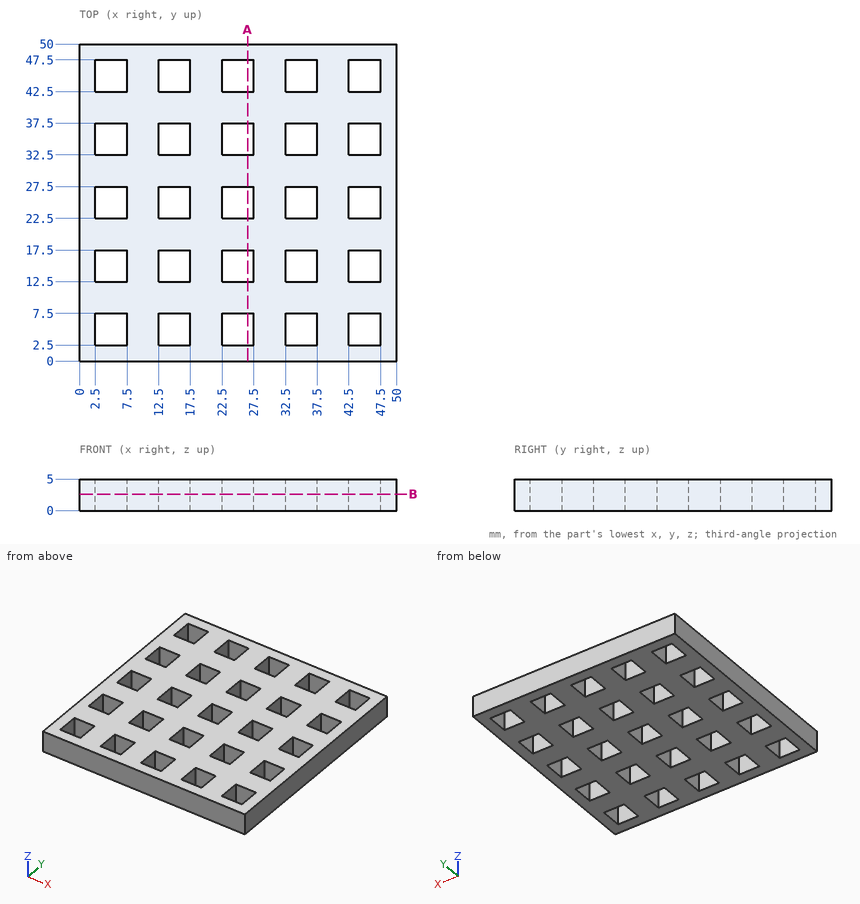
For this review, use the dimensioned drawing (mm, ordinates from the lowest corner) and the shaded views. Round coordinates to 2 decimals unless told otherwise and drop trailing zeros. Write each loop counter-clockwise with the first axis right and the second up, starting at its lowest first coordinate (ties: lowest second). Pieces come first, ordered by that corner, then holes. Notation, with made-up numbers: M 74.25,60.25 L 99.25,60.25 A20 cw 99.25,86.25 Z; hole C -1.5,-33.5 d11. An arc over 180 degrees is marked long. Write item = value, one per line. Start each with the question number.
(1) We need section B-B (z = 2.6). Give the number of separate pieces and of enclosed holes in the cut face, then the cut area to 4 significant figures.
(2) For line 1 along X through (y, z) = (46.5, 2.25), list the stretches that pass through material, from the lowest coordinate up.
(3) We need section A-A (x = 26.5). Give the boundary of the cut face in (y, z), then the cut area to 3 significant figures.
Results found:
q1.separate_pieces = 1
q1.enclosed_holes = 25
q1.area = 1,875 mm²
q2.line_1 = 0 to 2.5, 7.5 to 12.5, 17.5 to 22.5, 27.5 to 32.5, 37.5 to 42.5, 47.5 to 50
q3.outline = M 0,0 L 2.5,0 L 2.5,5 L 0,5 Z; M 7.5,0 L 12.5,0 L 12.5,5 L 7.5,5 Z; M 17.5,0 L 22.5,0 L 22.5,5 L 17.5,5 Z; M 27.5,0 L 32.5,0 L 32.5,5 L 27.5,5 Z; M 37.5,0 L 42.5,0 L 42.5,5 L 37.5,5 Z; M 47.5,0 L 50,0 L 50,5 L 47.5,5 Z
q3.area = 125 mm²
